Geometry: see drawing. Coordinates: mm, zero at the bounding-box minimum. A direction names the side the tool comes from. Round coordinates to 2 decimals unless told otherwise and drop trailing zeros. Loops run counter-clockwise (first coordinate to the right, second up) from the corner with the lowest first, then second, coordinate; pieces in that order, holes last. Notation, with made-up numbers: (61, 6) -> (101, 6) arc R9 cw to (101, 10) -> close; hole circle Ø3 at (70, 81.5). An arc over 180 degrees is marked (long way). Write item = value, one per line.
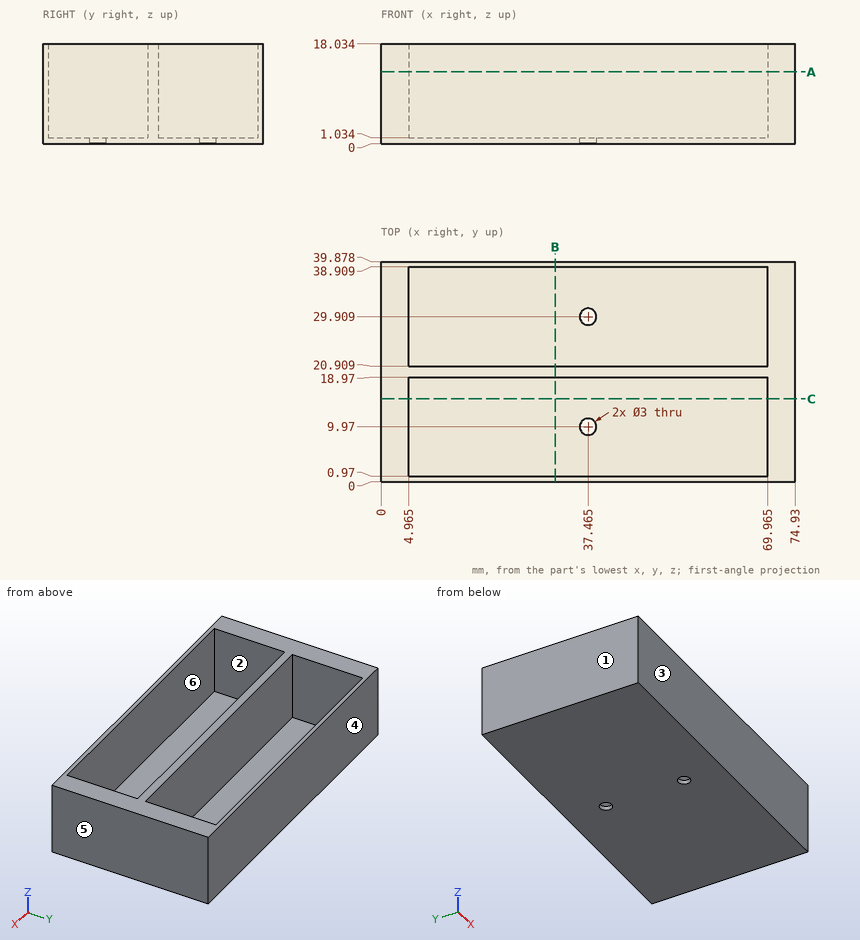
1. Section query C-C (y = 15). Return the cut outline in (x, z) (1 decimal).
Evaluation:
outline = (0, 0) -> (74.9, 0) -> (74.9, 18) -> (70, 18) -> (70, 1) -> (5, 1) -> (5, 18) -> (0, 18) -> close
2. Section query A-A (z = 13). Return the cut outline in (x, y) (1 decimal).
Evaluation:
outline = (0, 0) -> (74.9, 0) -> (74.9, 39.9) -> (0, 39.9) -> close; hole (5, 1) -> (70, 1) -> (70, 19) -> (5, 19) -> close; hole (5, 20.9) -> (70, 20.9) -> (70, 38.9) -> (5, 38.9) -> close
3. Set-up query: the marked faces 1 and 2. Return all of +Z, -Z, +X, -X, +Y, -Y with unobstructed straight access to the full face (end or side cutting, diameter ignored); none if empty.
Evaluation:
face_1 = +Z, -Z, -X, +Y, -Y
face_2 = +Z
4. Mould query, pull axis Y, two halves, no side actions, for the marked faces 3, 4, 5 and 6. Classes: released by +Y, released by -Y, zero draft, split by the parting line, or undercut.
Evaluation:
face_3 = released by -Y
face_4 = released by +Y
face_5 = zero draft
face_6 = undercut
5. Section query B-B (x = 31.5). Return the cut outline in (y, z) (1 decimal).
Evaluation:
outline = (0, 0) -> (39.9, 0) -> (39.9, 18) -> (38.9, 18) -> (38.9, 1) -> (20.9, 1) -> (20.9, 18) -> (19, 18) -> (19, 1) -> (1, 1) -> (1, 18) -> (0, 18) -> close
6. Contact query for a flat-ended pin moving along its axis: pin 1 Ø9 at (x, y) = (46, 28.5) entering from +Z. Output: stop coordinate, or through.
Evaluation:
pin_1 = 1.03
7. Line query: probe 1 along Y at (x, z) = (43, 14.25); probe 2 along X at (y, z) = (12.5, 15.25) (1 decimal); probe 3 along Z at (x, y) = (54.5, 27.5) (1 decimal). Output: solid intervals per line, ascending. Write a range as from..to.
Evaluation:
probe_1 = 0..0.97, 18.97..20.91, 38.91..39.88
probe_2 = 0..5, 70..74.9
probe_3 = 0..1
